For this review, take the finished solid that the model builds, in its own axes (mm). Give positions to 0.01 mm unless a question says otherwise; leave off trailing zeros. Order: outer loops, then holes, each group sorted by start corner. A loop starts at its lowest first (then second) coordinate and runs counter-clockwise, first axis right, second up. Notation, with made-up numbers: M -3.5,78 L 29.5,78 A19 cw 29.5,91 Z; hole C -19.5,12 d8. An arc over 180 degrees is marked long. Use CSV: the item, a comma, the result in double quotes. Start each with the question number.
(1) Wall thickness on L1, parallel to Y at x = 5.05, z = -14.5 (3 decimals); L2, parallel to Y at x = 4, z = -17 (3 decimals); L3, parallel to Z at x = 2.1, y = -75 (3 decimals): over which ranges is each line inside the solid? List them lowest first. Write a range as from..to.
(2) Consider section B-B (y = 11). Write out the cut boundary in (x, z) (3 decimals), and give its area (3 significant figures).
(3) Clearance check with flat-ended pins moving along their axes: P1, Ø1.5, axis at x = 2.5, y = 56.5, coming from the -Z side (3 decimals); P2, Ø1.7, axis at x = 3.5, z = -13, coming from the +Y side (3 decimals); P3, Ø3, axis at x = 2.5, y = 71.5, coming from the -Z side (3 decimals); P4, Ø2, axis at y = -61, z = 5.5, coming from the -X side. State where each tip first meets the part, or that it passes through.
(4) Consider section D-D (y = -57). Write out the cut boundary in (x, z) (3 decimals).
(5) Consider section A-A (z = -6). Give the number of separate pieces and of enclosed holes in the cut face, and give its area (3 significant figures).
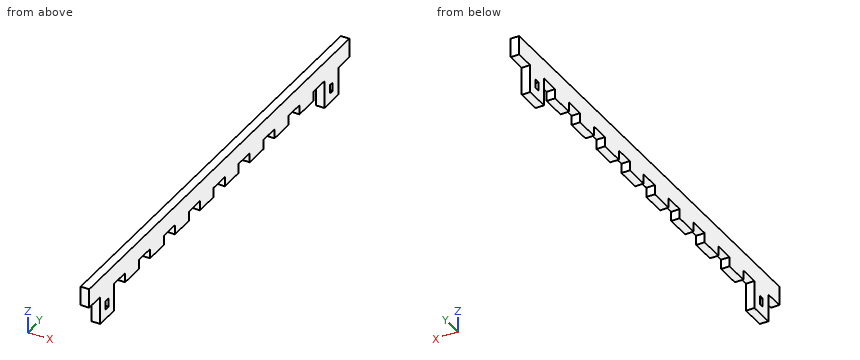
```python
from build123d import *

# Parameters (mm, degrees)
BOSS_EXTRUDE1_DEPTH = 5.588
BOSS_EXTRUDE2_DEPTH = 5.588


with BuildPart() as part:
    # Sketch1 → Boss-Extrude1 (new body)
    with BuildSketch(Plane(origin=(0, 0, 0), x_dir=(0, 0, -1), z_dir=(1, 0, 0))):
        Polygon((3.175, 120.65), (9.525, 120.65), (9.525, 136.525), (3.175, 136.525), (3.175, 149.225), (-9.525, 149.225), (-9.525, -149.225), (3.175, -149.225), (3.175, -136.525), (9.525, -136.525), (9.525, -120.65), (3.175, -120.65), (3.175, -107.95), (9.525, -107.95), (9.525, -92.075), (3.175, -92.075), (3.175, -79.375), (9.525, -79.375), (9.525, -63.5), (3.175, -63.5), (3.175, -50.8), (9.525, -50.8), (9.525, -34.925), (3.175, -34.925), (3.175, -22.225), (9.525, -22.225), (9.525, -6.35), (3.175, -6.35), (3.175, 6.35), (9.525, 6.35), (9.525, 22.225), (3.175, 22.225), (3.175, 34.925), (9.525, 34.925), (9.525, 50.8), (3.175, 50.8), (3.175, 63.5), (9.525, 63.5), (9.525, 79.375), (3.175, 79.375), (3.175, 92.075), (9.525, 92.075), (9.525, 107.95), (3.175, 107.95), align=None)
    extrude(amount=BOSS_EXTRUDE1_DEPTH)

    # Sketch2 → Boss-Extrude2 (add)
    with BuildSketch(Plane(origin=(5.588, 0, 0), x_dir=(0, 0, -1), z_dir=(1, 0, 0))):
        Polygon((21.717, -120.65), (9.525, -120.65), (9.525, -127), (15.367, -127), (15.367, -130.175), (9.525, -130.175), (9.525, -136.525), (21.717, -136.525), align=None)
        Polygon((21.717, 136.525), (9.525, 136.525), (9.525, 130.175), (15.367, 130.175), (15.367, 127), (9.525, 127), (9.525, 120.65), (21.717, 120.65), align=None)
    extrude(amount=-BOSS_EXTRUDE2_DEPTH)


solid = part.part
```
Check result:
1,L1,"y = -136.525..-130.175, -127..-120.65, 120.65..127, 130.175..136.525"
1,L2,"y = -136.525..-120.65, 120.65..136.525"
1,L3,"z = -9.525..9.525"
2,outline,"M 0,-9.525 L 5.588,-9.525 L 5.588,9.525 L 0,9.525 Z"
2,area,"106 mm^2"
3,P1,"stops at z = -3.175"
3,P2,"stops at y = 136.525"
3,P3,"stops at z = -9.525"
3,P4,"stops at x = 0"
4,outline,"M 0,-3.175 L 5.588,-3.175 L 5.588,9.525 L 0,9.525 Z"
5,separate pieces,"10"
5,enclosed holes,"0"
5,area,"887 mm^2"
